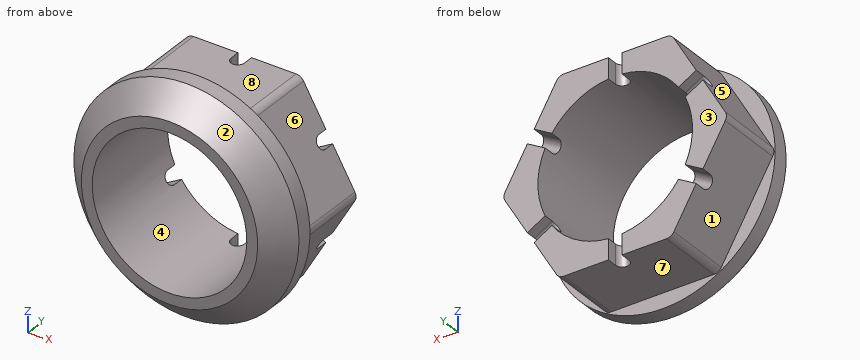
from build123d import *

# Parameters (mm, degrees)
CUT_EXTRUDE5_DEPTH = 20
FILLET4_R          = 2.5
CUT_EXTRUDE6_START = -62.5788381
CUT_EXTRUDE6_DEPTH = 96.5788382
CIRPATTERN2_COUNT  = 6


with BuildPart() as part:
    # Sketch1 → Revolve1 (revolve)
    with BuildSketch(Plane(origin=(0, 0, 0), x_dir=(0, 0, -1), z_dir=(1, 0, 0))):
        Polygon((-22.6695, -31.75), (-22.6695, 0), (-33, 0), (-33, -24.619433914), (-25.8445, -31.75), align=None)
    revolve(axis=Axis((0, 0, 0), (0, 1, 0)))

    # Sketch4 → Cut-Extrude5 (cut)
    with BuildSketch(Plane(origin=(0, 0, 0), x_dir=(1, 0, 0), z_dir=(0, 1, 0))):
        with BuildLine():
            ThreePointArc((33, 0), (28.578838325, 16.5), (16.5, 28.578838325))
            Line((16.5, 28.578838325), (33, 0))
        make_face()
        with BuildLine():
            Line((-16.5, 28.578838325), (16.5, 28.578838325))
            ThreePointArc((16.5, 28.578838325), (0, 33), (-16.5, 28.578838325))
        make_face()
        with BuildLine():
            Line((-33, 0), (-16.5, 28.578838325))
            ThreePointArc((-16.5, 28.578838325), (-28.578838325, 16.5), (-33, 0))
        make_face()
        with BuildLine():
            ThreePointArc((16.5, -28.578838325), (28.578838325, -16.5), (33, 0))
            Line((33, 0), (16.5, -28.578838325))
        make_face()
        with BuildLine():
            Line((-16.5, -28.578838325), (-33, 0))
            ThreePointArc((-33, 0), (-28.578838325, -16.5), (-16.5, -28.578838325))
        make_face()
        with BuildLine():
            ThreePointArc((-16.5, -28.578838325), (0, -33), (16.5, -28.578838325))
            Line((16.5, -28.578838325), (-16.5, -28.578838325))
        make_face()
    extrude(amount=-CUT_EXTRUDE5_DEPTH, mode=Mode.SUBTRACT)

    # Fillet4
    fillet4_edges = [part.edges().sort_by_distance(p)[0] for p in [
        (33, -10, 0),
        (16.5, -10, -28.578838325),
        (-33, -10, 0),
        (16.5, -10, 28.578838325),
        (-16.5, -10, -28.578838325),
        (-16.5, -10, 28.578838325),
    ]]
    fillet(fillet4_edges, radius=FILLET4_R)

    # Sketch7 → Cut-Extrude6 (cut)
    with BuildSketch(Plane.XY.offset(CUT_EXTRUDE6_START)):
        with BuildLine():
            Line((-1.984375, -3), (-1.984375, 0))
            Line((-1.984375, 0), (1.984375, 0))
            Line((1.984375, 0), (1.984375, -3))
            ThreePointArc((1.984375, -3), (0, -4.984375), (-1.984375, -3))
        make_face()
    cut_extrude6 = extrude(amount=CUT_EXTRUDE6_DEPTH, mode=Mode.SUBTRACT)

    # CirPattern2: Cut-Extrude6 ×6 about axis
    cirpattern2_axis = Axis((0, 0, 0), (0, 1, 0))
    for i in range(1, CIRPATTERN2_COUNT):
        add(cut_extrude6.rotate(cirpattern2_axis, i * 360 / CIRPATTERN2_COUNT), mode=Mode.SUBTRACT)


solid = part.part
Input: part model. Units: mm. Frame: model coordinates. Face numbers are marked on the shaded views. A direction names the side the tool comes from. Round coordinates to 2 decimals unless told otherwise and drop trailing zeros. Order: outer loops, then holes, each group sorted by start corner. A loop starts at its lowest first (then second) coordinate and runs counter-clockwise, first axis right, second up.
1. Set-up query: the marked faces 5, 6, 7 and 8. Return all of +Z, -Z, +X, -X, +Y, -Y with unobstructed straight access to the full face (end or side cutting, diameter ignored); none if empty.
The answers:
face 5: +Z, -X, +Y
face 6: +Z, +X, +Y
face 7: -Z, +X, -X, +Y
face 8: +Z, +X, -X, +Y
2. Mould query, pull axis X, two halves, no side actions, for the marked faces 1, 2, 3 and 4. Classes: released by +X, released by -X, zero draft, split by the parting line, or undercut.
The answers:
face 1: released by -X
face 2: split by the parting line
face 3: zero draft
face 4: undercut
3. Material intervals for line 1 (X direction, y = -15, z = 0); line 2 (Z direction, x = 0, y = -10); line 3 (X direction, y = -24, z = 0), sorted ascending.
The answers:
line 1: x = -32.61 to -22.67, 22.67 to 32.61
line 2: z = -28.58 to -22.67, 22.67 to 28.58
line 3: x = -33 to -22.67, 22.67 to 33
4. Cut plane A-A, the plane z = 0. Output: boundary loops of the cut face in (x, y).
The answers:
outline: (-33, -24.62) - (-25.84, -31.75) - (-22.67, -31.75) - (-22.67, 0) - (-32.61, 0) - (-32.61, -20) - (-33, -20) - close; (22.67, -31.75) - (25.84, -31.75) - (33, -24.62) - (33, -20) - (32.61, -20) - (32.61, 0) - (22.67, 0) - close
5. Cut plane C-C, the plane x = 0. Output: boundary loops of the cut face in (y, z), then the cut area to 3 significant figures.
The answers:
outline: (-31.75, -25.84) - (-24.62, -33) - (-20, -33) - (-20, -28.58) - (-4.98, -28.58) - (-4.98, -22.67) - (-31.75, -22.67) - close; (-31.75, 22.67) - (-4.98, 22.67) - (-4.98, 28.58) - (-20, 28.58) - (-20, 33) - (-24.62, 33) - (-31.75, 25.84) - close
area: 369 mm2
6. Pin query (flat end, axial travel): P1, Ø10, axis at x = 2.5, y = -13.5, coming from the +Z side; P2, Ø10, axis at x = 2.5, y = -9.5, coming from the -Z side; P3, Ø1, axis at x = -3, y = -21, coming from the -Z side; P4, Ø10, axis at x = 23, z = 2.5, coming from the +Y side. Return the tip coordinate at first contact, or that it passes through.
The answers:
P1: stops at z = 28.58
P2: stops at z = -28.58
P3: stops at z = -32.91
P4: stops at y = 0
7. Cut plane B-B, the plane y = -7.5. Output: boundary loops of the cut face in (x, z), then the cut area to 3 significant figures.
The answers:
outline: (-32.28, -1.25) - (-17.22, -27.33) arc R2.5 ccw to (-15.06, -28.58) - (15.06, -28.58) arc R2.5 ccw to (17.22, -27.33) - (32.28, -1.25) arc R2.5 ccw to (32.28, 1.25) - (17.22, 27.33) arc R2.5 ccw to (15.06, 28.58) - (-15.06, 28.58) arc R2.5 ccw to (-17.22, 27.33) - (-32.28, 1.25) arc R2.5 ccw to start; hole circle Ø45.34 at (0, 0)
area: 1,210 mm2
